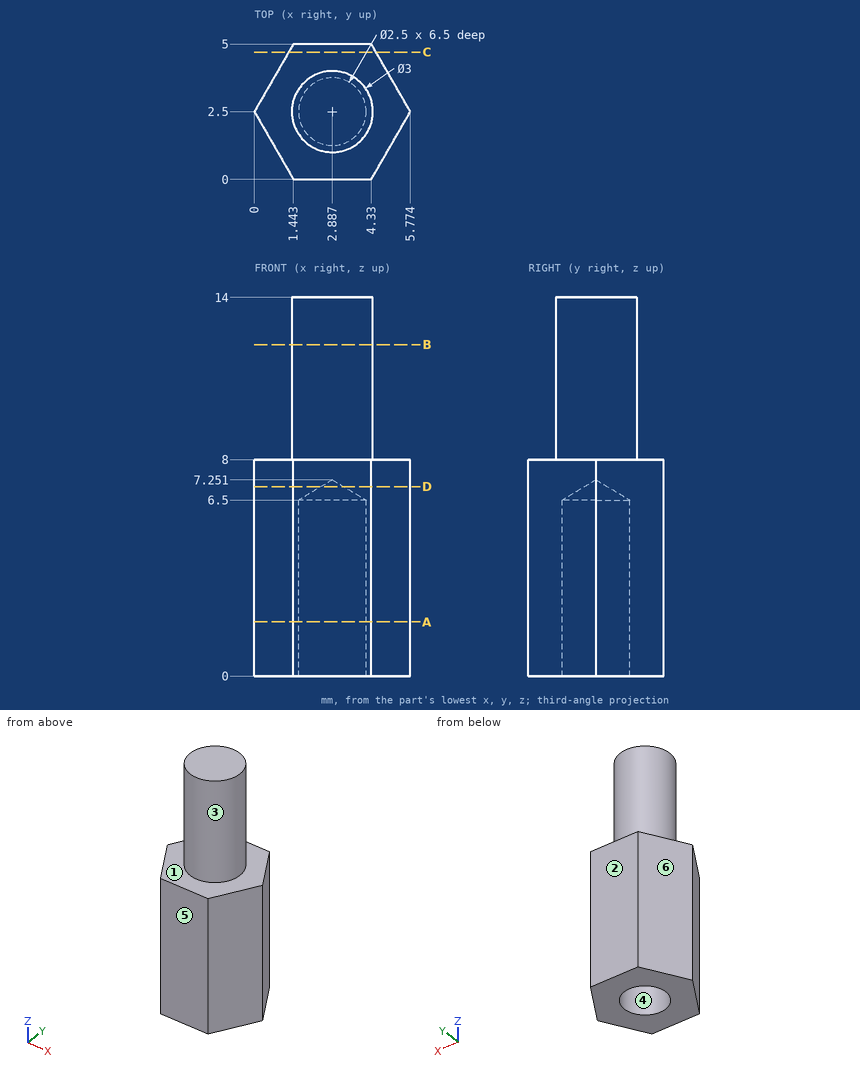
Here's the drawing with two shaded views (mm, measured from the low corner). I have some questions. A direction names the side the tool comes from. Give positions to 0.01 mm unless a question says otherwise; leave off trailing zeros. Loops run counter-clockwise (first coordinate to the right, second up) from the corner with the lowest first, then second, coordinate; pieces in that order, holes last. Notation, with made-up numbers: (65.5, -35.5) - (122.5, -35.5) arc R23 ccw to (122.5, -27.5) - close; hole circle Ø2 at (69, -18.5). An arc over 180 degrees is marked (long way). One line per item, written item: value.
(1) I need wall thicknesses on line 1 along Z through (x, y) = (1.85, 3.65); line 2 along X through (y, z) = (2.2, 2.25) (1 decimal); line 3 along X through (y, z) = (1.6, 1.5) (1 decimal). Which ranges of each line are inside material? Lowest first, please.
Verdict:
line 1: 0 to 8
line 2: 0.2 to 1.7, 4.1 to 5.6
line 3: 0.5 to 2, 3.8 to 5.3
(2) If we section it at C-C, the plane y = 4.7: List the corners of the cut face in (x, z) for me.
Verdict:
outline: (1.27, 0) - (4.5, 0) - (4.5, 8) - (1.27, 8) - close
(3) If we mould it in two halves opening along X, with no side actions, what happens to the marked faces 3, 4, 5 and 6? For each: released by +X, released by -X, zero draft, split by the parting line, or undercut.
Verdict:
face 3: split by the parting line
face 4: undercut
face 5: zero draft
face 6: released by -X
(4) I'm going to push flat-ended pins straight in: pin 1 (2 mm diameter, centred on y = 3.5, z = 11.5, fed in from -X); pin 2 (1.5 mm diameter, centred on y = 1, z = 8, fed in from +X); pin 3 (2 mm diameter, centred on x = 4.5, z = 6, fed in from -Y). Where does each tip first touch, or does it pass through?
Verdict:
pin 1: x = 1.39
pin 2: x = 5.34
pin 3: y = 0
(5) On a 3-axis mill with a long thin cutter (end or side, diameter ignored), from which of +Z, -Z, +X, -X, +Y, -Y can I reach the whole of each face in a straight line? I mean the marked faces 1 and 2. Say none if no direction works.
Verdict:
face 1: +Z
face 2: +Z, -Z, +X, -X, +Y
(6) If we section it at D-D, the plane z = 7: List the corners of the cut face in (x, y) for me (1 decimal).
Verdict:
outline: (0, 2.5) - (1.4, 0) - (4.3, 0) - (5.8, 2.5) - (4.3, 5) - (1.4, 5) - close; hole circle Ø0.8 at (2.9, 2.5)
(7) If we section it at B-B, the plane z = 12.25: List the corners of the cut face in (x, y) for me.
Verdict:
outline: circle Ø3 at (2.89, 2.5)
(8) If we section it at A-A, the plane z = 2: List the corners of the cut face in (x, y) for me.
Verdict:
outline: (0, 2.5) - (1.44, 0) - (4.33, 0) - (5.77, 2.5) - (4.33, 5) - (1.44, 5) - close; hole circle Ø2.5 at (2.89, 2.5)
